Read the model definition and answer for the solid it produces. Units are mm, in the model's axes. A direction names the side the tool comes from. Round coordinates to 2 decimals unless told otherwise and drop trailing zeros. Write each loop counter-clockwise with the first axis right and the second up, starting at its lowest first coordinate (ties: lowest second). Pieces come first, ordered by that corner, then holes. Notation, with made-up numbers: (52.25, -7) - (65.25, -7) arc R34 cw to (65.25, 29) - close; hole circle Ø8 at (40.25, -25.75). An arc over 180 degrees is marked (long way). Use one line per item in the form item = value. Start each with the question number.
1) The part is cut by section C-C, the plane z = -7. Count the separate pieces of the cut face and the enclosed holes in it, plus the area to 3 significant figures.
2) The part is cut by section A-A, the plane x = 0. Give the vertices of the cut face in (y, z).
3) For faces 1 (the face through (21.62, -1.77, 6.05)), 2 (the face through (-18.8, 1.2, -5.4)), 3 (the face through (-17.6, -2, -9)), 4 (the face through (-18, 0, -28)), determine the directions among +Z, -Z, +X, -X, +Y, -Y from which every point of the face is accessible in a straight line to the end or side of a thin tool.
4) Each of these flat-tipped pins is pushed along its axis until it touches: pin 1 (2.5 mm diameter, centred on y = 0, z = 21.5, fed in from -X); pin 2 (6.5 mm diameter, centred on y = 0, z = -21.5, fed in from +X); pin 3 (1.5 mm diameter, centred on x = -8.5, y = 0, fed in from +Z); pin 4 (3 mm diameter, centred on y = 0, z = 7, fed in from -X). Where does it stop, or does it pass through?
5) For a pull along Y with two mould halves and no side action, classify faces 5 (the face through (-18.23, -6.93, 27.4)), 6 (the face through (17.26, -0.72, -8.68)), 7 (the face through (13.77, -0.11, 13.63)), 8 (the face through (-17.6, -2, 5)) as released by +Y, released by -Y, zero draft, split by the parting line, or undercut.
6) Consider line 1 along Z through (x, y) = (-19.15, 0); line 2 along Y through (x, z) = (-18.25, 7); line 3 along X through (y, z) = (-3, 19). Determine where each line is inside the solid, lowest interval first. Write a range as from..to.
7) The part is cut by section D-D, the plane x = 9.5. Give the vertices of the cut face in (y, z).
from build123d import *

# Parameters (mm, degrees)
BOSS_EXTRUDE1_DEPTH               = 7.5
BOSS_EXTRUDE1_DEPTH_BACK          = 7.5
SKETCH4_W                         = 2
SKETCH4_H                         = 4
F_4_0_4_DIAMETER_HOLE1_AT_2_COUNT = 2
F_4_0_4_DIAMETER_HOLE1_AT_2_PITCH = 43
F_4_0_4_DIAMETER_HOLE1_AT_3_COUNT = 2
F_4_0_4_DIAMETER_HOLE1_AT_3_PITCH = 14.5
F_4_0_4_DIAMETER_HOLE1_AT_4_COUNT = 2
F_4_0_4_DIAMETER_HOLE1_AT_4_PITCH = 28.5
FILLET1_R                         = 2
CUT_EXTRUDE1_DEPTH                = 1
CUT_EXTRUDE5_REACH                = 52.268
CUT_EXTRUDE5_END_RADIUS           = 16
SKETCH15_R                        = 3.5
CUT_EXTRUDE5_DIRECTION_2_DEPTH    = 0.6
FILLET2_R                         = 0.5
BOSS_EXTRUDE2_START               = -7.5
BOSS_EXTRUDE2_DEPTH               = 15
CUT_EXTRUDE6_REACH                = 45.576
SKETCH17_R                        = 2
CUT_EXTRUDE7_REACH                = 45.576


with BuildPart() as part:
    # Sketch1 → Boss-Extrude1 (new, two sides: drawn at the far end of the back side and taken through both)
    with BuildSketch(Plane(origin=(0, 0, 0), x_dir=(1, 0, 0), z_dir=(0, 1, 0)).offset(-BOSS_EXTRUDE1_DEPTH_BACK)):
        with BuildLine():
            Line((-16, 14.966629547), (-16, 28))
            Line((-16, 28), (-20, 28))
            Line((-20, 28), (-20, -28))
            Line((-20, -28), (-16, -28))
            Line((-16, -28), (-16, -14.966629547))
            Line((-16, -14.966629547), (-10, -14.966629547))
            ThreePointArc((-10, -14.966629547), (4.335878308, -17.469978801), (15.837588826, -8.553992061))
            Line((15.837588826, -8.553992061), (23.80714641, -9.251238003))
            Line((23.80714641, -9.251238003), (24.068613639, -6.262653909))
            Line((24.068613639, -6.262653909), (15.035081933, -5.472322293))
            ThreePointArc((15.035081933, -5.472322293), (-16, 0), (15.035081933, 5.472322293))
            Line((15.035081933, 5.472322293), (24.068613639, 6.262653909))
            Line((24.068613639, 6.262653909), (23.80714641, 9.251238003))
            Line((23.80714641, 9.251238003), (15.837588826, 8.553992061))
            ThreePointArc((15.837588826, 8.553992061), (4.335878308, 17.469978801), (-10, 14.966629547))
            Line((-10, 14.966629547), (-16, 14.966629547))
        make_face()
    extrude(amount=BOSS_EXTRUDE1_DEPTH + BOSS_EXTRUDE1_DEPTH_BACK)

    # Sketch4 → Ø4.0 (4) Diameter Hole1 (revolve, cut)
    with BuildSketch(Plane(origin=(-16, 0, 21.5), x_dir=(0, 0, -1), z_dir=(0, 1, 0))):
        with Locations((1, 2)):
            Rectangle(SKETCH4_W, SKETCH4_H)
    f_4_0_4_diameter_hole1 = revolve(axis=Axis((-9.65, 0, 21.5), (-1, 0, 0)), mode=Mode.SUBTRACT)

    # Ø4.0 (4) Diameter Hole1 at 2: Ø4.0 (4) Diameter Hole1 ×2
    with Locations(*[(0, 0, -i * F_4_0_4_DIAMETER_HOLE1_AT_2_PITCH) for i in range(1, F_4_0_4_DIAMETER_HOLE1_AT_2_COUNT)]):
        add(f_4_0_4_diameter_hole1, mode=Mode.SUBTRACT)

    # Ø4.0 (4) Diameter Hole1 at 3: Ø4.0 (4) Diameter Hole1 ×2
    with Locations(*[(0, 0, -i * F_4_0_4_DIAMETER_HOLE1_AT_3_PITCH) for i in range(1, F_4_0_4_DIAMETER_HOLE1_AT_3_COUNT)]):
        add(f_4_0_4_diameter_hole1, mode=Mode.SUBTRACT)

    # Ø4.0 (4) Diameter Hole1 at 4: Ø4.0 (4) Diameter Hole1 ×2
    with Locations(*[(0, 0, -i * F_4_0_4_DIAMETER_HOLE1_AT_4_PITCH) for i in range(1, F_4_0_4_DIAMETER_HOLE1_AT_4_COUNT)]):
        add(f_4_0_4_diameter_hole1, mode=Mode.SUBTRACT)

    # Fillet1
    fillet1_edges = [part.edges().sort_by_distance(p)[0] for p in [
        (-18, -7.5, -28),
        (-18, -7.5, 28),
        (-18, 7.5, -28),
        (-18, 7.5, 28),
    ]]
    fillet(fillet1_edges, radius=FILLET1_R)

    # Sketch10 → Cut-Extrude1 (cut)
    with BuildSketch(Plane(origin=(-16, 0, 0), x_dir=(0, 0, -1), z_dir=(1, 0, 0))):
        with BuildLine():
            Line((14.966629547, 6), (14.966629547, -6))
            Line((14.966629547, -6), (26, -6))
            ThreePointArc((26, -6), (26.353553391, -5.853553391), (26.5, -5.5))
            Line((26.5, -5.5), (26.5, 5.5))
            ThreePointArc((26.5, 5.5), (26.353553391, 5.853553391), (26, 6))
            Line((26, 6), (14.966629547, 6))
        make_face()
        with BuildLine():
            Line((-14.966629547, 6), (-14.966629547, -6))
            Line((-14.966629547, -6), (-26, -6))
            ThreePointArc((-26, -6), (-26.353553391, -5.853553391), (-26.5, -5.5))
            Line((-26.5, -5.5), (-26.5, 5.5))
            ThreePointArc((-26.5, 5.5), (-26.353553391, 5.853553391), (-26, 6))
            Line((-26, 6), (-14.966629547, 6))
        make_face()
    extrude(amount=-CUT_EXTRUDE1_DEPTH, mode=Mode.SUBTRACT)

    # Cut-Extrude5: up to this cylinder (the profile starts outside it)
    cut_extrude5_end = Plane(origin=(0, 0, 0), z_dir=(0, 1, 0)) * Cylinder(CUT_EXTRUDE5_END_RADIUS, 137.536, mode=Mode.PRIVATE)
    # Sketch15 → Cut-Extrude5 (cut, up to the surface)
    with BuildSketch(Plane(origin=(-17, 0, 0), x_dir=(0, 0, -1), z_dir=(1, 0, 0)), mode=Mode.PRIVATE) as cut_extrude5_sk1:
        with Locations((7, 0)):
            Circle(SKETCH15_R)
    cut_extrude5_tool1 = extrude(cut_extrude5_sk1.sketch, amount=CUT_EXTRUDE5_REACH, mode=Mode.PRIVATE) - cut_extrude5_end
    add(cut_extrude5_tool1.solids().sort_by_distance((-17, 0, -7))[0], mode=Mode.SUBTRACT)
    # Sketch15 → Cut-Extrude5 (cut, up to the surface)
    with BuildSketch(Plane(origin=(-17, 0, 0), x_dir=(0, 0, -1), z_dir=(1, 0, 0)), mode=Mode.PRIVATE) as cut_extrude5_sk2:
        with Locations((-7, 0)):
            Circle(SKETCH15_R)
    cut_extrude5_tool2 = extrude(cut_extrude5_sk2.sketch, amount=CUT_EXTRUDE5_REACH, mode=Mode.PRIVATE) - cut_extrude5_end
    add(cut_extrude5_tool2.solids().sort_by_distance((-17, 0, 7))[0], mode=Mode.SUBTRACT)

    # Sketch15 → Cut-Extrude5 direction 2 (cut)
    with BuildSketch(Plane(origin=(-17, 0, 0), x_dir=(0, 0, -1), z_dir=(1, 0, 0))):
        with Locations((7, 0)):
            Circle(SKETCH15_R)
        with Locations((-7, 0)):
            Circle(SKETCH15_R)
    extrude(amount=-CUT_EXTRUDE5_DIRECTION_2_DEPTH, mode=Mode.SUBTRACT)

    # Fillet2
    fillet2_edges = [part.edges().sort_by_distance(p)[0] for p in [
        (-17, -6, -20.483314774),
        (-17, -5.853553391, -26.353553391),
        (-17, 0, -26.5),
        (-17, 5.853553391, -26.353553391),
        (-16, -6, -20.483314774),
        (-16, -5.853553391, -26.353553391),
        (-16, 6, -20.483314774),
        (-16, 5.853553391, -26.353553391),
        (-16, -7.5, -20.483314774),
        (-16, -6.914213562, -27.414213562),
        (-16, 7.5, -20.483314774),
        (-16, 6.914213562, -27.414213562),
        (-16, -7.5, 20.483314774),
        (-16, -6.914213562, 27.414213562),
        (-16, 0, 28),
        (-16, 6.914213562, 27.414213562),
        (-17, -6, 20.483314774),
        (-17, -5.853553391, 26.353553391),
        (-17, 0, 26.5),
        (-17, 5.853553391, 26.353553391),
        (-16, -6, 20.483314774),
        (-16, -5.853553391, 26.353553391),
        (-16, 0, 26.5),
        (-16, 5.853553391, 26.353553391),
        (-17, 6, -20.483314774),
        (-16, 0, -26.5),
        (-16, 0, -28),
        (-16, 7.5, 20.483314774),
        (-17, 6, 20.483314774),
        (-16, 6, 20.483314774),
    ]]
    fillet(fillet2_edges, radius=FILLET2_R - 0.0001)  # a hair under: the kernel refuses the full size

    # Sketch11 → Boss-Extrude2 (add)
    with BuildSketch(Plane(origin=(0, 0, 0), x_dir=(1, 0, 0), z_dir=(0, 1, 0)).offset(BOSS_EXTRUDE2_START)):
        with BuildLine():
            Line((23.80714641, -9.251238003), (7.198399175, -16.497971066))
            ThreePointArc((7.198399175, -16.497971066), (12.183631905, -13.24987221), (15.837588826, -8.553992061))
            Line((15.837588826, -8.553992061), (23.80714641, -9.251238003))
        make_face()
        with BuildLine():
            Line((23.80714641, 9.251238003), (7.198399175, 16.497971066))
            ThreePointArc((7.198399175, 16.497971066), (12.183631905, 13.24987221), (15.837588826, 8.553992061))
            Line((15.837588826, 8.553992061), (23.80714641, 9.251238003))
        make_face()
    extrude(amount=BOSS_EXTRUDE2_DEPTH)

    # Sketch16 → Cut-Revolve1 (revolve, cut)
    with BuildSketch(Plane(origin=(0, 0, 0), x_dir=(1, 0, 0), z_dir=(0, 1, 0)), mode=Mode.PRIVATE) as cut_revolve1_sk:
        Polygon((19.551847786, -5.867488101), (21.544237182, -6.041799587), (21.282769954, -9.030383681), (23.026110675, -9.182906231), (22.079695592, -20.000480134), (18.343965474, -19.673646099), align=None)
    revolve(cut_revolve1_sk.sketch.rotate(Axis((19.551847786, 0, 5.867488101), (-0.08715574274765382, 0, 0.996194698091746)), 180), axis=Axis((19.551847786, 0, 5.867488101), (-0.08715574274765382, 0, 0.996194698091746)), mode=Mode.SUBTRACT)

    # Sketch17 → Cut-Extrude6 (cut, up to next)
    with BuildSketch(Plane(origin=(-0.622388286, 0, -7.113930662), x_dir=(0.996194698091746, 0, -0.08715574274765478), z_dir=(0.08715574274765478, 0, 0.996194698091746)), mode=Mode.PRIVATE) as cut_extrude6_sk1:
        with Locations((19.988832385, 0)):
            Circle(SKETCH17_R)
    cut_extrude6_tool1 = extrude(cut_extrude6_sk1.sketch, amount=CUT_EXTRUDE6_REACH, mode=Mode.PRIVATE) & part.part
    add(cut_extrude6_tool1.solids().sort_by_distance((19.290381, 0, -8.856072))[0], mode=Mode.SUBTRACT)

    # Cut-Extrude7: up to this plane
    cut_extrude7_end = Plane(origin=(23.80714641, -25.910792681, -9.251238003), z_dir=(0.39991106530273124, 0, -0.9165539481385887))
    # Sketch18 → Cut-Extrude7 (cut, up to the surface)
    with BuildSketch(Plane(origin=(-0.622388286, 0, -7.113930662), x_dir=(0.996194698091746, 0, -0.08715574274765478), z_dir=(0.08715574274765478, 0, 0.996194698091746)), mode=Mode.PRIVATE) as cut_extrude7_sk1:
        Polygon((16.988832385, -1.732050808), (19.988832385, -3.464101615), (22.988832385, -1.732050808), (22.988832385, 1.732050808), (19.988832385, 3.464101615), (16.988832385, 1.732050808), align=None)
    cut_extrude7_tool1 = split(extrude(cut_extrude7_sk1.sketch, amount=-CUT_EXTRUDE7_REACH, mode=Mode.PRIVATE), bisect_by=cut_extrude7_end, keep=Keep.BOTH, mode=Mode.PRIVATE)
    add(cut_extrude7_tool1.solids().sort_by_distance((19.290381, 0, -8.856072))[0], mode=Mode.SUBTRACT)


solid = part.part
Geometry results:
q1.separate_pieces = 3
q1.enclosed_holes = 1
q1.area = 184 mm2
q2.outline = (-7.5, -18) - (7.5, -18) - (7.5, -16) - (-7.5, -16) - close; (-7.5, 16) - (7.5, 16) - (7.5, 18) - (-7.5, 18) - close
q3.face_1 = +X, +Y, -Y
q3.face_2 = -X
q3.face_3 = none
q3.face_4 = -Z, +X, -X, +Y, -Y
q4.pin_1 = through
q4.pin_2 = -17
q4.pin_3 = 16.25
q4.pin_4 = 13.56
q5.face_5 = released by -Y
q5.face_6 = undercut
q5.face_7 = zero draft
q5.face_8 = undercut
q6.line_1 = -28..-23.5, -19.5..-9, -5..5, 9..19.5, 23.5..28
q6.line_2 = -7.5..-2, 2..7.5
q6.line_3 = -20..-17
q7.outline = (-7.5, -15.49) - (7.5, -15.49) - (7.5, -12.87) - (-7.5, -12.87) - close; (-7.5, 12.87) - (7.5, 12.87) - (7.5, 15.49) - (-7.5, 15.49) - close
